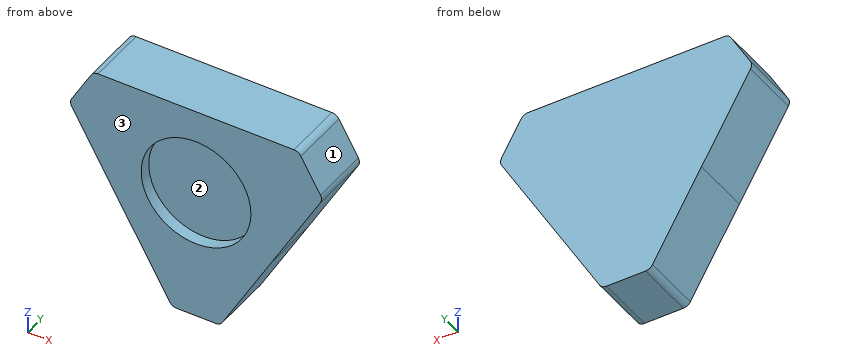
```python
from build123d import *

# Parameters (mm, degrees)
SKETCH2_R               = 21.650635095
BOSS_EXTRUDE1_DEPTH     = 15
CUT_EXTRUDE1_DEPTH      = 1
CUT_EXTRUDE1_DEPTH_BACK = 16
FILLET1_R               = 2
SKETCH4_R               = 13.650635095
CUT_EXTRUDE2_DEPTH      = 3


with BuildPart() as part:
    # Sketch2 → Boss-Extrude1 (new body)
    with BuildSketch(Plane(origin=(0, 0, 0), x_dir=(1, 0, 0), z_dir=(0, 1, 0))):
        with Locations((37.5, 21.650635095)):
            Circle(SKETCH2_R)
        with BuildLine():
            Line((18.749999007, 32.475950921), (0, 0))
            Line((0, 0), (37.5, 0))
            ThreePointArc((37.5, 0), (18.750000497, 10.825316687), (18.749999007, 32.475950921))
        make_face()
        with BuildLine():
            Line((37.5, 64.951905284), (18.749999007, 32.475950921))
            ThreePointArc((18.749999007, 32.475950921), (37.499999914, 43.301270189), (56.250000907, 32.47595107))
            Line((56.250000907, 32.47595107), (37.5, 64.951905284))
        make_face()
        with BuildLine():
            ThreePointArc((59.150635095, 21.650635095), (52.809310892, 6.341324202), (37.5, 0))
            Line((37.5, 0), (75, 0))
            Line((75, 0), (56.250000907, 32.47595107))
            ThreePointArc((56.250000907, 32.47595107), (58.412907828, 27.254230919), (59.150635095, 21.650635095))
        make_face()
    extrude(amount=BOSS_EXTRUDE1_DEPTH)

    # Sketch3 → Cut-Extrude1 (cut, two sides)
    with BuildSketch(Plane(origin=(0, 15, 0), x_dir=(1, 0, 0), z_dir=(0, 1, 0))) as cut_extrude1_sk:
        Polygon((31.5, 54.559600438), (43.5, 54.559600438), (37.5, 64.951905284), align=None)
        Polygon((0, 0), (6, 10.392304845), (12, 0), align=None)
        Polygon((75, 0), (69, 10.392304845), (63, 0), align=None)
    extrude(amount=CUT_EXTRUDE1_DEPTH, mode=Mode.SUBTRACT)
    extrude(cut_extrude1_sk.sketch, amount=-CUT_EXTRUDE1_DEPTH_BACK, mode=Mode.SUBTRACT)

    # Fillet1
    fillet1_edges = [part.edges().sort_by_distance(p)[0] for p in [
        (31.5, 7.5, -54.559600438),
        (43.5, 7.5, -54.559600438),
        (12, 7.5, 0),
        (6, 7.5, -10.392304845),
        (63, 7.5, 0),
        (69, 7.5, -10.392304845),
    ]]
    fillet(fillet1_edges, radius=FILLET1_R)

    # Sketch4 → Cut-Extrude2 (cut)
    with BuildSketch(Plane.XZ):
        with Locations((37.5, -21.650635095)):
            Circle(SKETCH4_R)
    extrude(amount=-CUT_EXTRUDE2_DEPTH, mode=Mode.SUBTRACT)


solid = part.part
```
Read the model definition and answer for the solid it produces. Units are mm, in the model's axes. Face numbers are marked on the shaded views. Coordinates: 2 decimals unless noted, no trailing zeros. Loops run counter-clockwise (first coordinate to the right, second up) from the corner with the lowest first, then second, coordinate; pieces in that order, holes last.
(1) The part is cut by section D-D (y = 1.5). Determine the outline of the cut face in (x, z), and give its area (3 significant figures).
Solution:
outline: (6.58, -11.39) - (30.92, -53.56) arc R2 ccw to (32.65, -54.56) - (42.35, -54.56) arc R2 ccw to (44.08, -53.56) - (68.42, -11.39) arc R2 ccw to (68.42, -9.39) - (63.58, -1) arc R2 ccw to (61.85, 0) - (13.15, 0) arc R2 ccw to (11.42, -1) - (6.58, -9.39) arc R2 ccw to start; hole circle Ø27.3 at (37.5, -21.65)
area: 1,660 mm2
(2) Flat-ended cylindrical pins translate along their axes: pin 1 Ø5 at (x, y) = (19.5, 12.5) entering from -Z; pin 2 Ø6 at (x, y) = (53.5, 4.5) entering from -Z; pin 3 Ø6 at (y, z) = (5.5, -24) entering from +X. Find the tip coordinate at first contact, or state that the pin passes through.
Solution:
pin 1: stops at z = -38.11
pin 2: stops at z = -42.44
pin 3: stops at x = 62.88
(3) The part is cut by section A-A (x = 37.5). Determine the outline of the cut face in (y, z), and give its area (3 significant figures).
Solution:
outline: (0, -54.56) - (15, -54.56) - (15, 0) - (0, 0) - (0, -8) - (3, -8) - (3, -35.3) - (0, -35.3) - close
area: 736 mm2
(4) The part is cut by section C-C (z = -17). Determine the outline of the cut face in (x, y), and give its area (3 significant figures).
Solution:
outline: (9.81, 0) - (24.67, 0) - (24.67, 3) - (50.33, 3) - (50.33, 0) - (65.19, 0) - (65.19, 15) - (9.81, 15) - close
area: 754 mm2
(5) Consider line 1 along Z through (x, y) = (37.5, 1.15); line 2 along X through (y, z) = (2.75, -26); line 3 along Y through (x, z) = (35, -11). Determine where each line is inside the solid, lowest interval first.
Solution:
line 1: z = -54.56 to -35.3, -8 to 0
line 2: x = 15.01 to 24.56, 50.44 to 59.99
line 3: y = 3 to 15
(6) The mould has two halves that part along Z. Classify the marked faces 1, 2 and 3: released by +Z, released by -Z, zero draft, split by the parting line, or undercut.
Solution:
face 1: released by +Z
face 2: undercut
face 3: zero draft
(7) The part is cut by section B-B (y = 7.5). Determine the outline of the cut face in (x, z).
Solution:
outline: (6.58, -11.39) - (30.92, -53.56) arc R2 ccw to (32.65, -54.56) - (42.35, -54.56) arc R2 ccw to (44.08, -53.56) - (68.42, -11.39) arc R2 ccw to (68.42, -9.39) - (63.58, -1) arc R2 ccw to (61.85, 0) - (13.15, 0) arc R2 ccw to (11.42, -1) - (6.58, -9.39) arc R2 ccw to start
